Verification items for the finished model (mm, model axes). Round coordinates to 2 decimals unless told otherwise and drop trailing zeros. Order: outer loops, then holes, each group sorted by start corner. A loop starts at its lowest first (then second) coordinate and runs counter-clockwise, first axis right, second up. Notation, with made-up numbers: M 85.25,41 L 101.25,41 A17 cw 101.25,72 Z; hole C 88.5,-28.75 d3. An arc over 180 degrees is marked long. Use CSV: the item, a comma, the result in double quotes. Start each with the question number.
Q1. Sectioned sample at C-C (y = 0.15). State how many separate pieces and enclosed holes the cut face has, and give its area (3 significant figures).
Q2. Sectioned sample at A-A (x = -99.5). Enter the section's corners in (y, z).
Q3. Scan lines: line 1 (Z direction, x = 37.5, y = 1.45); line 2 (Z direction, x = 94.5, y = -0.3); line 3 (X direction, y = 1.2, z = 38). Record each from-to range of solid material in increasing order.
Q4. Sectioned sample at B-B (z = 99). Enter the section's corners in (x, y).
Q5. Gauge pin test, flat ends, axial feed: pin 1 Ø3 at (x, z) = (24, -31) entering from -Y; pin 2 Ø1 at (x, y) = (77, 1) entering from -Z; pin 3 Ø1 at (x, y) = (0.5, 1) entering from -Z. Record the tip position at first contact, or that the pin passes through.
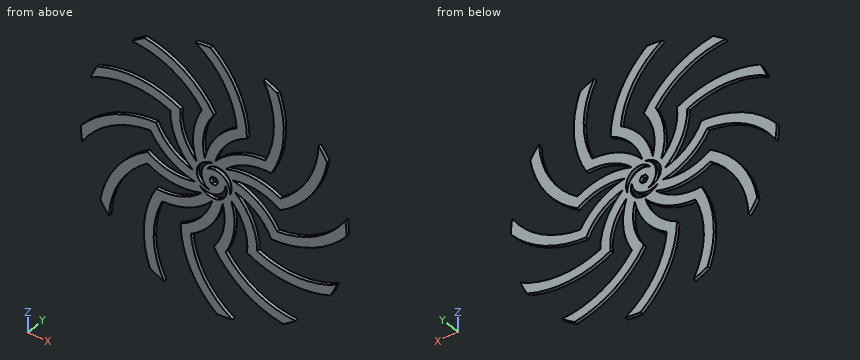
```python
from build123d import *

# Parameters (mm, degrees)
BOSS_EXTRUDE1_DEPTH = 1
CIRPATTERN1_COUNT   = 12
SKETCH2_R           = 6.32456178
BOSS_EXTRUDE2_DEPTH = 1
CUT_EXTRUDE1_DEPTH  = 57.561097513
SCALE1_SCALE        = 3.4
CUT_EXTRUDE2_DEPTH  = 3.4


with BuildPart() as part:
    # Sketch1 → Boss-Extrude1 (new body)
    with BuildSketch(Plane(origin=(0, 0, 0), x_dir=(1, 0, 0), z_dir=(0, 1, 0))):
        with BuildLine():
            ThreePointArc((0, 20), (3.252272915, 10), (0, 0))
            Line((0, 0), (3.572780991, 0))
            ThreePointArc((3.572780991, 0), (6.252272915, 10), (3.572780991, 20))
            ThreePointArc((3.572780991, 20), (12.742280623, 28.230711371), (24.614013417, 31.530149754))
            ThreePointArc((24.614013417, 31.530149754), (22.757477342, 32.895246238), (20.825411836, 34.151167211))
            ThreePointArc((20.825411836, 34.151167211), (8.856268151, 29.366098374), (0, 20))
        make_face()
    extrude(amount=BOSS_EXTRUDE1_DEPTH)


with BuildPart() as cirpattern1_1:
    # CirPattern1: pattern copy
    add(part.part.rotate(Axis((0, 0, 0), (0, 1, 0)), 1 * 360 / CIRPATTERN1_COUNT))


with BuildPart() as cirpattern1_2:
    # CirPattern1: pattern copy
    add(part.part.rotate(Axis((0, 0, 0), (0, 1, 0)), 2 * 360 / CIRPATTERN1_COUNT))


with BuildPart() as cirpattern1_3:
    # CirPattern1: pattern copy
    add(part.part.rotate(Axis((0, 0, 0), (0, 1, 0)), 3 * 360 / CIRPATTERN1_COUNT))


with BuildPart() as cirpattern1_4:
    # CirPattern1: pattern copy
    add(part.part.rotate(Axis((0, 0, 0), (0, 1, 0)), 4 * 360 / CIRPATTERN1_COUNT))


with BuildPart() as cirpattern1_5:
    # CirPattern1: pattern copy
    add(part.part.rotate(Axis((0, 0, 0), (0, 1, 0)), 5 * 360 / CIRPATTERN1_COUNT))


with BuildPart() as cirpattern1_6:
    # CirPattern1: pattern copy
    add(part.part.rotate(Axis((0, 0, 0), (0, 1, 0)), 6 * 360 / CIRPATTERN1_COUNT))


with BuildPart() as cirpattern1_7:
    # CirPattern1: pattern copy
    add(part.part.rotate(Axis((0, 0, 0), (0, 1, 0)), 7 * 360 / CIRPATTERN1_COUNT))


with BuildPart() as cirpattern1_8:
    # CirPattern1: pattern copy
    add(part.part.rotate(Axis((0, 0, 0), (0, 1, 0)), 8 * 360 / CIRPATTERN1_COUNT))


with BuildPart() as cirpattern1_9:
    # CirPattern1: pattern copy
    add(part.part.rotate(Axis((0, 0, 0), (0, 1, 0)), 9 * 360 / CIRPATTERN1_COUNT))


with BuildPart() as cirpattern1_10:
    # CirPattern1: pattern copy
    add(part.part.rotate(Axis((0, 0, 0), (0, 1, 0)), 10 * 360 / CIRPATTERN1_COUNT))


with BuildPart() as cirpattern1_11:
    # CirPattern1: pattern copy
    add(part.part.rotate(Axis((0, 0, 0), (0, 1, 0)), 11 * 360 / CIRPATTERN1_COUNT))


with BuildPart() as part_1:
    add(part.part)

    add(cirpattern1_1.part)  # Boss-Extrude2 merges CirPattern1_1

    add(cirpattern1_2.part)  # Boss-Extrude2 merges CirPattern1_2

    add(cirpattern1_3.part)  # Boss-Extrude2 merges CirPattern1_3

    add(cirpattern1_4.part)  # Boss-Extrude2 merges CirPattern1_4

    add(cirpattern1_5.part)  # Boss-Extrude2 merges CirPattern1_5

    add(cirpattern1_6.part)  # Boss-Extrude2 merges CirPattern1_6

    add(cirpattern1_7.part)  # Boss-Extrude2 merges CirPattern1_7

    add(cirpattern1_8.part)  # Boss-Extrude2 merges CirPattern1_8

    add(cirpattern1_9.part)  # Boss-Extrude2 merges CirPattern1_9

    add(cirpattern1_10.part)  # Boss-Extrude2 merges CirPattern1_10

    add(cirpattern1_11.part)  # Boss-Extrude2 merges CirPattern1_11
    # Sketch2 → Boss-Extrude2 (add)
    with BuildSketch(Plane(origin=(0, 0, 0), x_dir=(1, 0, 0), z_dir=(0, 1, 0))):
        Circle(SKETCH2_R)
    extrude(amount=BOSS_EXTRUDE2_DEPTH)

    # Sketch3 → Cut-Extrude1 (cut, through all)
    with BuildSketch(Plane(origin=(0, 1, 0), x_dir=(1, 0, 0), z_dir=(0, 1, 0))):
        with BuildLine():
            ThreePointArc((-0.518779192, -5.29922884), (-3.404124769, -2.355249802), (-3.031088913, 1.75))
            ThreePointArc((-3.031088913, 1.75), (-2.338245241, 2.604344292), (-1.414452319, 3.201456643))
            ThreePointArc((-1.414452319, 3.201456643), (-4.658051165, 1.166519136), (-4.611205766, -2.66228089))
            ThreePointArc((-4.611205766, -2.66228089), (-2.884018037, -4.47586842), (-0.518779192, -5.29922884))
        make_face()
        with BuildLine():
            ThreePointArc((3.5, 0), (3.494938576, -0.188160443), (3.479768941, -0.375776681))
            ThreePointArc((3.479768941, -0.375776681), (3.339260789, 3.450731073), (0, 5.32456178))
            ThreePointArc((0, 5.32456178), (-2.434206737, 4.735567095), (-4.3298772, 3.098890379))
            ThreePointArc((-4.3298772, 3.098890379), (-0.337643776, 4.125683429), (3.031088913, 1.75))
            ThreePointArc((3.031088913, 1.75), (3.380740392, 0.905866658), (3.5, 0))
        make_face()
        with BuildLine():
            ThreePointArc((0, -3.5), (-1.086305696, -3.327151925), (-2.065316622, -2.825679962))
            ThreePointArc((-2.065316622, -2.825679962), (1.318790377, -4.617250209), (4.611205766, -2.66228089))
            ThreePointArc((4.611205766, -2.66228089), (5.143131737, -1.378097996), (5.32456178, 0))
            ThreePointArc((5.32456178, 0), (5.204225623, 1.1256082), (4.848656392, 2.200338461))
            ThreePointArc((4.848656392, 2.200338461), (3.741768545, -1.770433627), (0, -3.5))
        make_face()
    extrude(amount=-CUT_EXTRUDE1_DEPTH, mode=Mode.SUBTRACT)


with BuildPart() as part_2:
    # Scale1: scaled about (0, 0.5, 0)
    add(part_1.part.scale(SCALE1_SCALE).moved(Location((0, -1.2, 0))))

    # Sketch4 → Cut-Extrude2 (cut)
    with BuildSketch(Plane(origin=(0, 2.2, 0), x_dir=(1, 0, 0), z_dir=(0, 1, 0))):
        Polygon((-4.35, 0), (-2.175, -3.767210506), (2.175, -3.767210506), (4.35, 0), (2.175, 3.767210506), (-2.175, 3.767210506), align=None)
    extrude(amount=-CUT_EXTRUDE2_DEPTH, mode=Mode.SUBTRACT)


solid = part_2.part
```
Verdict:
1,separate pieces,"1"
1,enclosed holes,"4"
1,area,"18,200 mm²"
2,outline,"M -1.2,-50.46 L 2.2,-50.46 L 2.2,-29.61 L -1.2,-29.61 Z; M -1.2,13.45 L 2.2,13.45 L 2.2,24.8 L -1.2,24.8 Z; M -1.2,60.07 L 2.2,60.07 L 2.2,70.42 L -1.2,70.42 Z"
3,line 1,"z = -104.42 to -92.51, -60.74 to -22.73, -8.97 to 2.82, 10.95 to 21.17, 32.25 to 42.77"
3,line 2,"z = -71.09 to -60.82, -26.92 to -15.86, 22.94 to 40.72"
3,line 3,"x = -42.89 to -32.39, -21.14 to -10.92, -2.56 to 9.3, 23.76 to 60.99, 92.83 to 104.7"
4,outline,"M -49.34,-1.2 L -28.89,-1.2 L -28.89,2.2 L -49.34,2.2 Z; M 13.71,-1.2 L 25.02,-1.2 L 25.02,2.2 L 13.71,2.2 Z; M 60.16,-1.2 L 70.5,-1.2 L 70.5,2.2 L 60.16,2.2 Z"
5,pin 1,"passes through"
5,pin 2,"stops at z = -112.44"
5,pin 3,"stops at z = -134.05"
